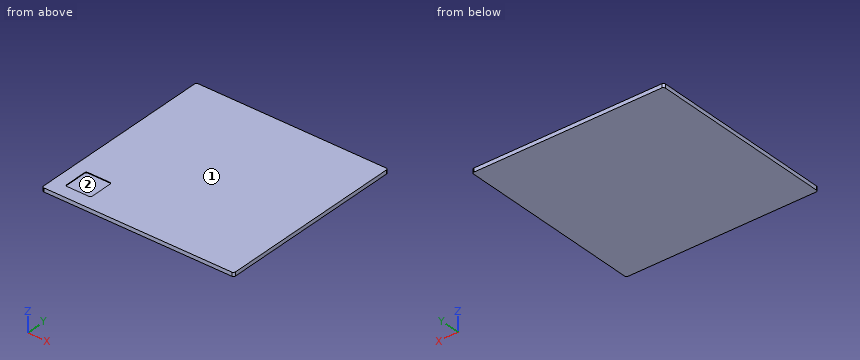
Autodesk Inventor part; units mm, degrees
ref_plane "YZ Plane" through (0, 0, 0) normal (1, 0, 0) x (0, 1, 0)
ref_plane "XZ Plane" through (0, 0, 0) normal (0, 1, 0) x (-1, 0, 0)
ref_plane "XY Plane" through (0, 0, 0) normal (0, 0, 1) x (1, 0, 0)
sketch "Sketch1" plane through (0, 0, 0) normal (0, 0, 1) x (1, 0, 0)
  line L0 (-150, -148) -> (150, -148)
  line L1 (150, -148) -> (150, 148)
  line L2 (150, 148) -> (-150, 148)
  line L3 (-150, 148) -> (-150, -148)
  line L4 (-150, -148) -> (150, 148) construction
  line L5 (150, -148) -> (-150, 148) construction
  point P0 (0, 0)
  dimension "d0" = 296
  dimension "d1" = 300
extrude "Extrusion1" add sketch "Sketch1" along normal blind 6
sketch "Sketch2" plane through (0, 0, 6) normal (0, 0, 1) x (1, 0, 0)
  line L0 (-130, -128) -> (-90, -128)
  line L1 (-90, -128) -> (-90, -88)
  line L2 (-90, -88) -> (-130, -88)
  line L3 (-130, -88) -> (-130, -128)
  line L4 (-150, 148) -> (-150, -148)
  line L5 (-150, -148) -> (150, -148)
  point P0 (0, 0)
  dimension "d4" = 20
  dimension "d5" = 20
  dimension "d6" = 40
  dimension "d7" = 40
extrude "Extrusion2" cut sketch "Sketch2" against normal blind 1
fillet "Fillet1" radius 3 4 edges at (-130, -88, 5.5) (-90, -88, 5.5) (-90, -128, 5.5) (-130, -128, 5.5)
fillet "Fillet2" radius 3 4 edges at (-150, -148, 3) (150, -148, 3) (150, 148, 3) (-150, 148, 3)
equation "\"d5\" = d4"
properties part number "VacuumTableAdjustmentPlate"
Part model, mm, in its own coordinate system. Face numbers are marked on the shaded views. Give positions to 0.01 mm unless a question says otherwise; leave off trailing zeros. Order: outer loops, then holes, each group sorted by start corner. A loop starts at its lowest first (then second) coordinate and runs counter-clockwise, first axis right, second up. Notation, with made-up numbers: M -9,1 L 29,1 A32 ccw 29,37 Z; hole C -24.5,53 d5. An arc over 180 degrees is marked long. Use a Markdown table: item, result. Add a question column.
(1) Probe line 1 along Y through (x, z) = (-101, 5.6). List the from-to ranges inside material, lowest first. Write a range as [from, to].
(2) Saw through at A-A, the plane y = -102. Give the cut face in (x, z).
(3) Mould opens along X. For the marked faces 1 and 2 say: +X half, -X half, draft (parallel to the pull), parting line (faces both ways), or undercut.
(4) Drop a flat-ended pin along its axis: P1, Ø20, axis at x = -107, y = -108, coming from the +Z side. Give the stop position or say it passes through.
Answer key:
| question | item | result |
|---|---|---|
| 1 | line 1 | [-148, -128], [-88, 148] |
| 2 | outline | M -150,0 L 150,0 L 150,6 L -90,6 L -90,5 L -130,5 L -130,6 L -150,6 Z |
| 3 | face 1 | draft |
| 3 | face 2 | undercut |
| 4 | P1 | z = 5 |
